CAD build for the part. Positions are in the model's coordinates, mm. A direction names the side the tool comes from. Round coordinates to 2 decimals unless told otherwise and drop trailing zeros. Loops run counter-clockwise (first coordinate to the right, second up) from the corner with the lowest first, then second, coordinate; pieces in that order, holes last. Notation, with made-up numbers: M 1.25,70 L 11.25,70 A33 ccw 11.25,107 Z; hole C 83.25,10.25 d2. An arc over 180 degrees is marked long. Use a Markdown table: item, result. Add a question column.
(1) Band-saw the part on C-C, the plane z = 0. Write the cut outline in (x, y).
(2) Which spindle directions (+Z, -Z, +X, -X, +Y, -Y) get a long thin tool onto all of the face, cutting with end or side? Do faces 1 (the face through (-25, 44, 0)), 2 (the face through (25, 44, 0)), 3 (the face through (2, 18, -2)), 4 (the face through (2.04, 22, 0.99)). Say none if no direction does.
(3) Two-plate mould, pull along Z, no slides. Class faces 5 (the face through (-2.29, 8.87, 5.91)), 6 (the face through (-1, 44, 13)), 7 (the face through (8, 40, 8)): released by +Z, released by -Z, zero draft, split by the parting line, or undercut.
(4) Band-saw the part on A-A, the plane y = 44. Give the number of separate pieces and of enclosed holes in the cut face, and give its area (3 significant figures).
(5) Wall check: L1, parallel to X at y = 20.5, z = 0; L2, parallel to Y at x = -33.45, z = 10. Give the ranges that are in metal, low to high.
(6) Band-saw the part on B-B, the plane x = 33.45. Write the cut outline in (y, z) (3 decimals), and give its area (3 significant figures).
(7) Flat gauge pins, fed straight in: P1, Ø6, axis at y = 25.5, z = 6.5, coming from the -X side; P2, Ø1, axis at y = 42, z = -5.5, coming from the -X side; P3, Ø7.5, axis at x = 0, z = 0, coming from the +Y side. Where does each tip first touch, or does it go through?
(8) Band-saw the part on D-D, the plane y = 8.5. Write the cut outline in (x, z), and give its area (3 significant figures).
from build123d import *

# Parameters (mm, degrees)
SKETCH_10_R         = 10.85
EXTRUDE_5_DEPTH     = 40
CUT_EXTRUDE_1_DEPTH = 18
SKETCH_12_R         = 4.75
CUT_EXTRUDE_2_DEPTH = 18
SKETCH_13_R         = 2.1
CUT_EXTRUDE_3_DEPTH = 4
SKETCH_14_W         = 76
SKETCH_14_H         = 26
EXTRUDE_8_DEPTH     = 8
SKETCH_15_R         = 4.75
CUT_EXTRUDE_4_DEPTH = 8
SKETCH_16_R         = 1.6
CUT_EXTRUDE_5_DEPTH = 26
SKETCH_17_W         = 13
SKETCH_17_H         = 12.15
CUT_EXTRUDE_6_DEPTH = 8


with BuildPart() as part:
    # 草图10 → 凸台-拉伸5 (new body)
    with BuildSketch(Plane(origin=(0, 0, 0), x_dir=(1, 0, 0), z_dir=(0, 1, 0))):
        Circle(SKETCH_10_R)
    extrude(amount=EXTRUDE_5_DEPTH)

    # 草图11 → 切除-拉伸1 (cut)
    with BuildSketch(Plane(origin=(0, 0, 0), x_dir=(-1, 0, 0), z_dir=(0, -1, 0))):
        Polygon((5.739953665, -4.542612896), (6.803995, 2.699639243), (1.064041335, 7.242252139), (-5.739953665, 4.542612896), (-6.803995, -2.699639243), (-1.064041335, -7.242252139), align=None)
    extrude(amount=-CUT_EXTRUDE_1_DEPTH, mode=Mode.SUBTRACT)

    # 草图12 → 切除-拉伸2 (cut)
    with BuildSketch(Plane(origin=(0, 40, 0), x_dir=(1, 0, 0), z_dir=(0, 1, 0))):
        Circle(SKETCH_12_R)
    extrude(amount=-CUT_EXTRUDE_2_DEPTH, mode=Mode.SUBTRACT)

    # 草图13 → 切除-拉伸3 (cut)
    with BuildSketch(Plane(origin=(0, 22, 0), x_dir=(1, 0, 0), z_dir=(0, 1, 0))):
        Circle(SKETCH_13_R)
    extrude(amount=-CUT_EXTRUDE_3_DEPTH, mode=Mode.SUBTRACT)

    # 草图14 → 凸台-拉伸8 (add)
    with BuildSketch(Plane(origin=(0, 40, 0), x_dir=(1, 0, 0), z_dir=(0, 1, 0))):
        Rectangle(SKETCH_14_W, SKETCH_14_H)
    extrude(amount=EXTRUDE_8_DEPTH)

    # 草图15 → 切除-拉伸4 (cut)
    with BuildSketch(Plane(origin=(0, 48, 0), x_dir=(1, 0, 0), z_dir=(0, 1, 0))):
        Circle(SKETCH_15_R)
    extrude(amount=-CUT_EXTRUDE_4_DEPTH, mode=Mode.SUBTRACT)

    # 草图16 → 切除-拉伸5 (cut)
    with BuildSketch(Plane.XY.offset(13)):
        with Locations((-33.45, 44)):
            Circle(SKETCH_16_R)
        with Locations((33.45, 44)):
            Circle(SKETCH_16_R)
    extrude(amount=-CUT_EXTRUDE_5_DEPTH, mode=Mode.SUBTRACT)

    # 草图17 → 切除-拉伸6 (cut)
    with BuildSketch(Plane.XZ.offset(-40)):
        with Locations((31.5, 0)):
            Rectangle(SKETCH_17_W, SKETCH_17_H)
        with Locations((-31.5, 0)):
            Rectangle(SKETCH_17_W, SKETCH_17_H)
    extrude(amount=-CUT_EXTRUDE_6_DEPTH, mode=Mode.SUBTRACT)


solid = part.part
Return value:
| question | item | result |
|---|---|---|
| 1 | outline | M -25,40 L -10.85,40 L -10.85,0 L -6.41,0 L -6.41,18 L -2.1,18 L -2.1,22 L -4.75,22 L -4.75,48 L -25,48 Z; M 2.1,18 L 6.41,18 L 6.41,0 L 10.85,0 L 10.85,40 L 25,40 L 25,48 L 4.75,48 L 4.75,22 L 2.1,22 Z |
| 2 | face 1 | -X, +Y, -Y |
| 2 | face 2 | +X, +Y, -Y |
| 2 | face 3 | -Y |
| 2 | face 4 | +Y |
| 3 | face 5 | undercut |
| 3 | face 6 | released by +Z |
| 3 | face 7 | zero draft |
| 4 | separate pieces | 5 |
| 4 | enclosed holes | 1 |
| 4 | area | 1,500 mm^2 |
| 5 | L1 | -10.85 to -2.1, 2.1 to 10.85 |
| 5 | L2 | 40 to 42.4, 45.6 to 48 |
| 6 | outline | M 40,-13 L 42.4,-13 L 42.4,-6.075 L 40,-6.075 Z; M 40,6.075 L 42.4,6.075 L 42.4,13 L 40,13 Z; M 45.6,-13 L 48,-13 L 48,-6.075 L 45.6,-6.075 Z; M 45.6,6.075 L 48,6.075 L 48,13 L 45.6,13 Z |
| 6 | area | 66.5 mm^2 |
| 7 | P1 | x = -10.27 |
| 7 | P2 | x = -25 |
| 7 | P3 | y = 22 |
| 8 | outline | C 0,0 d21.7; hole M -6.8,-2.7 L -1.06,-7.24 L 5.74,-4.54 L 6.8,2.7 L 1.06,7.24 L -5.74,4.54 Z |
| 8 | area | 231 mm^2 |
